For this review, take the finished solid that the model builds, in its own axes (mm). Face numbers are marked on the shaded views. A direction names the side the tool comes from. Coordinates: 2 decimals unless noted, no trailing zeros. Order: outer loops, then holes, each group sorted by start corner. A loop starts at its lowest first (then second) coordinate and runs counter-clockwise, first axis right, second up. Notation, with made-up numbers: (3, -31.75) - (16, -31.75) arc R37 ccw to (16, 5.25) - close; hole circle Ø10 at (24, 86.25). An arc over 180 degrees is marked (long way). One line per item, written item: value. Start each with the question number.
(1) Consider section C-C on y = -5.5. Count the separate pieces of the cut face and the enclosed holes in it, then the cut area to 3 significant figures.
(2) Consider section D-D on z = 90.5. Write out the cut boundary in (x, y).
(3) To check wall thickness, follow line 1 along X through (y, z) = (16.5, 62); line 2 along Y through (x, z) = (50, -9.5); line 3 along X through (y, z) = (-6, -4.5). State the ranges of each line that lie inside material, in increasing order.
(4) Mouldability with a two-part tool opening along Z and no side actions: class the marked faces 4, 5, 6 and 7 as released by +Z, released by -Z, zero draft, split by the parting line, or undercut.
(5) Clearance check with flat-ended pins moving along their axes: pin 1 (3 mm diameter, centred on x = 21.5, z = 57, fed in from -Y); pin 2 (12 mm diameter, centred on x = 4.5, z = -7.5, fed in from -Y); pin 3 (5 mm diameter, centred on y = 6.5, z = 101, fed in from +X); pin 4 (16.5 mm diameter, centred on x = 27.5, z = -7, fed in from +Y). State where each tip first meets the part, or that it passes through.
(6) Consider section A-A on x = -50. Write out the cut boundary in (y, z), then the cut area to 3 significant figures.
(7) For the marked faces 1, 2 and 3, list the 3-axis set-ups (+Z, -Z, +X, -X, +Y, -Y) from which the entire face can be reached by the end or side of a thin tool; tool diameter is ignored.
(8) Consider section B-B on z = 34. Write out the cut boundary in (x, y), then the cut area to 3 significant figures.
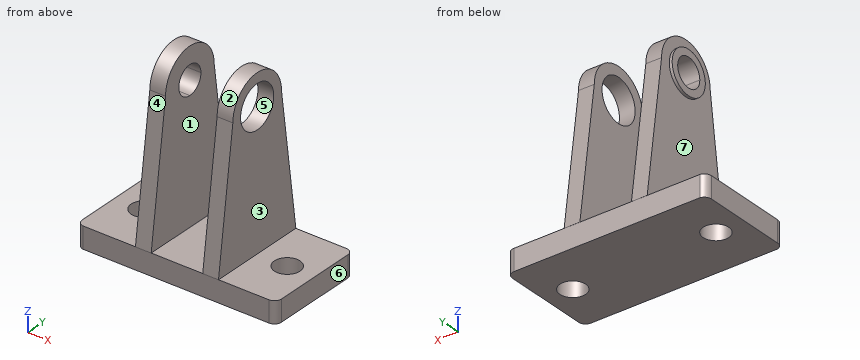
```python
from build123d import *

# Parameters (mm, degrees)
F5_DEPTH = 15
F6_DEPTH = 11
F7_DEPTH = 11
F8_DEPTH = 13


# Not quite as in the source:
# - a feature of the source that left no trace in its solid (it failed there, or was rolled back) is left out


with BuildPart() as f5:
    # F0 (on Top) → F5 (new body)
    with BuildSketch(Plane.XY):
        with BuildLine():
            Line((-70, 30), (-70, 0))
            Line((-70, 0), (-70, -30))
            ThreePointArc((-70, -30), (-68.8225510753, -33.2230580629), (-65.8447586893, -34.9281216256))
            Line((-65.8447586893, -34.9281216256), (64.1552413107, -34.9281216256))
            ThreePointArc((64.1552413107, -34.9281216256), (67.6652703796, -33.4889776935), (69.154724634, -30))
            Line((69.154724634, -30), (69.154724634, 0))
            Line((69.154724634, 0), (69.154724634, 30))
            ThreePointArc((69.154724634, 30), (67.6652703796, 33.4889776935), (64.1552413107, 34.9281216256))
            Line((64.1552413107, 34.9281216256), (-65.8447586893, 34.9281216256))
            ThreePointArc((-65.8447586893, 34.9281216256), (-68.8225510753, 33.2230580629), (-70, 30))
        make_face()
        with BuildLine():
            ThreePointArc((-41, 0), (-50, -9), (-59, 0))
            ThreePointArc((-59, 0), (-50, 9), (-41, 0))
        make_face(mode=Mode.SUBTRACT)
        with BuildLine():
            ThreePointArc((59, 0), (50, -9), (41, 0))
            ThreePointArc((41, 0), (50, 9), (59, 0))
        make_face(mode=Mode.SUBTRACT)
    extrude(amount=-F5_DEPTH)

    # F2 (on offset) → F6 (join)
    with BuildSketch(Plane.YZ.offset(-18)):
        with BuildLine():
            Line((-35, 0), (0, 0))
            Line((0, 0), (35, 0))
            Line((35, 0), (22, 95))
            ThreePointArc((22, 95), (0, 117), (-22, 95))
            Line((-22, 95), (-35, 0))
        make_face()
        with BuildLine():
            ThreePointArc((15, 95), (10.6066017178, 84.3933982822), (0, 80))
            ThreePointArc((0, 80), (-10.6066017178, 84.3933982822), (-15, 95))
            ThreePointArc((-15, 95), (0, 110), (15, 95))
        make_face(mode=Mode.SUBTRACT)
    extrude(amount=-F6_DEPTH)

    # F4 (on offset) → F7 (join)
    with BuildSketch(Plane.YZ.offset(18)):
        with BuildLine():
            ThreePointArc((22, 95), (0, 117), (-22, 95))
            Line((-22, 95), (-35, 0))
            Line((-35, 0), (0, 0))
            Line((0, 0), (35, 0))
            Line((35, 0), (22, 95))
        make_face()
        with BuildLine():
            ThreePointArc((15, 95), (10.6066017178, 84.3933982822), (0, 80))
            ThreePointArc((0, 80), (-10.6066017178, 84.3933982822), (-15, 95))
            ThreePointArc((-15, 95), (0, 110), (15, 95))
        make_face(mode=Mode.SUBTRACT)
    extrude(amount=F7_DEPTH)

    # F2 (on offset) → F8 (join)
    with BuildSketch(Plane.YZ.offset(-18)):
        with BuildLine():
            ThreePointArc((-15, 95), (-10.6066017178, 84.3933982822), (0, 80))
            ThreePointArc((0, 80), (10.6066017178, 84.3933982822), (15, 95))
            ThreePointArc((15, 95), (0, 110), (-15, 95))
        make_face()
        with BuildLine():
            ThreePointArc((10, 95), (7.0710678119, 87.9289321881), (0, 85))
            ThreePointArc((0, 85), (-7.0710678119, 87.9289321881), (-10, 95))
            ThreePointArc((-10, 95), (0, 105), (10, 95))
        make_face(mode=Mode.SUBTRACT)
    extrude(amount=-F8_DEPTH)


solid = f5.part
```
Geometry check:
1. separate pieces: 5
1. enclosed holes: 0
1. area: 3,750 mm^2
2. outline: (-31, -14.31) - (-29, -14.31) - (-29, -22.62) - (-18, -22.62) - (-18, -8.93) - (-31, -8.93) - close; (-31, 8.93) - (-18, 8.93) - (-18, 22.62) - (-29, 22.62) - (-29, 14.31) - (-31, 14.31) - close; (18, -22.62) - (29, -22.62) - (29, -14.31) - (18, -14.31) - close; (18, 14.31) - (29, 14.31) - (29, 22.62) - (18, 22.62) - close
3. line 1: x = -29 to -18, 18 to 29
3. line 2: y = -34.93 to -9, 9 to 34.93
3. line 3: x = -70 to -56.71, -43.29 to 43.29, 56.71 to 69.15
4. face 4: released by +Z
4. face 5: undercut
4. face 6: zero draft
4. face 7: undercut
5. pin 1: stops at y = -27.41
5. pin 2: stops at y = -34.93
5. pin 3: stops at x = -18
5. pin 4: stops at y = 35
6. outline: (-34.93, -15) - (-9, -15) - (-9, 0) - (-34.93, 0) - close; (9, -15) - (34.93, -15) - (34.93, 0) - (9, 0) - close
6. area: 778 mm^2
7. face 1: +Z, +Y, -Y
7. face 2: +Z, +X, -X
7. face 3: +Z, +X, +Y, -Y
8. outline: (-29, -30.35) - (-18, -30.35) - (-18, 30.35) - (-29, 30.35) - close; (18, -30.35) - (29, -30.35) - (29, 30.35) - (18, 30.35) - close
8. area: 1,340 mm^2
